Check sheet for the modelled part. Datum: model origin and axes. Units: mm. A direction names the side the tool comes from. Give positions to 0.01 mm unless a question says otherwise; leave off trailing zeros. Order: outer loops, then holes, each group sorted by start corner. A loop starts at its lowest first (then second) coordinate and runs counter-clockwise, first axis right, second up. Notation, with made-up numbers: (-40, -32) -> (-12, -32) arc R23 ccw to (-12, 6) -> close; hole circle Ø11 at (68.5, 36.25). An arc over 180 degrees is marked (long way). One line per question, with ' | ' between items.
```python
from build123d import *

# Parameters (mm, degrees)
CYLINDER_R           = 2.15
CYLINDER_DEPTH       = 50
CYLINDER_PITCH_ANGLE = 90
BOX002_W             = 14
BOX002_H             = 11
BOX002_DEPTH         = 20.5
CHAMFER_SIZE         = 4
FILLET001_R          = 5
BOX003_W             = 14
BOX003_H             = 25
BOX003_DEPTH         = 4
BOX003_ROLL_ANGLE    = -15
BOX004_W             = 14
BOX004_H             = 2.5
BOX004_DEPTH         = 5
POCKET006_DEPTH      = 15
BOX005003_W          = 42
BOX005003_H          = 6
BOX005003_DEPTH      = 25
SKETCH009_R          = 11
SKETCH009_R_2        = 1.75
POCKET009_DEPTH      = 6
SKETCH010_W          = 62.382877
SKETCH010_H          = 25.148186
POCKET010_DEPTH      = 6
BOX005002_W          = 13.8
BOX005002_H          = 6
BOX005002_DEPTH      = 42
CHAMFER002_SIZE      = 13
FILLET003_R          = 4
FILLET004_R          = 2
SKETCH011_R          = 2.95
POCKET011_DEPTH      = 4


with BuildPart() as cylinder:
    # Cylinder → Cylinder (new body)
    with BuildSketch(Plane.XY):
        Circle(CYLINDER_R)
    extrude(amount=CYLINDER_DEPTH)


with BuildPart() as cylinder_1:
    # Cylinder pitch: moved
    add(cylinder.part.rotate(Axis((0, 0, 0), (0, 1, 0)), CYLINDER_PITCH_ANGLE))


with BuildPart() as cylinder_2:
    # Cylinder placement: moved
    add(cylinder_1.part.moved(Location((31, -6, 12.9))))


with BuildPart() as fillet001:
    # Box002 → Box002 (new body)
    with BuildSketch(Plane(origin=(52, -12, -3), x_dir=(1, 0, 0), z_dir=(0, 0, 1))):
        with Locations((7, 5.5)):
            Rectangle(BOX002_W, BOX002_H)
    extrude(amount=BOX002_DEPTH)

    # Chamfer
    chamfer_edges = [fillet001.edges().sort_by_distance(p)[0] for p in [
        (59, -1, -3),
    ]]
    chamfer(chamfer_edges, length=CHAMFER_SIZE)

    # Fillet001
    fillet001_edges = [fillet001.edges().sort_by_distance(p)[0] for p in [
        (59, -1, 17.5),
    ]]
    fillet(fillet001_edges, radius=FILLET001_R)


with BuildPart() as cube002:
    # Box003 → Box003 (new body)
    with BuildSketch(Plane.XY):
        with Locations((7, 12.5)):
            Rectangle(BOX003_W, BOX003_H)
    extrude(amount=BOX003_DEPTH)


with BuildPart() as cube002_1:
    # Box003 roll: moved
    add(cube002.part.rotate(Axis((0, 0, 0), (1, 0, 0)), BOX003_ROLL_ANGLE))


with BuildPart() as cube002_2:
    # Box003 placement: moved
    add(cube002_1.part.moved(Location((52, -12, -3))))


with BuildPart() as obj1:
    # Box004 → Box004 (new body)
    with BuildSketch(Plane(origin=(52, -12, 14), x_dir=(1, 0, 0), z_dir=(0, 0, 1))):
        with Locations((7, 1.25)):
            Rectangle(BOX004_W, BOX004_H)
    extrude(amount=BOX004_DEPTH)

    # Fusion: union Fillet001, Cube002
    add(fillet001.part)
    add(cube002_2.part)

    # Cut001: cut Cylinder
    add(cylinder_2.part, mode=Mode.SUBTRACT)

    # Sketch006 → Pocket006 (cut)
    with BuildSketch(Plane.YZ.offset(66)):
        Polygon((13.183422, -5.606773), (-4.041064, -0.991486), (-0.407217, 12.570217), align=None)
    extrude(amount=-POCKET006_DEPTH, mode=Mode.SUBTRACT)


with BuildPart() as pocket010:
    # Box005003 → Box005003 (new body)
    with BuildSketch(Plane(origin=(52.2, -15.5, -42), x_dir=(1, 0, 0), z_dir=(0, 0, 1))):
        with Locations((21, 3)):
            Rectangle(BOX005003_W, BOX005003_H)
    extrude(amount=BOX005003_DEPTH)

    # Sketch009 → Pocket009 (cut)
    with BuildSketch(Plane(origin=(52.2, -9.5, -42), x_dir=(-1, 0, 0), z_dir=(0, 1, 0))):
        with Locations((-21, 1.5)):
            Circle(SKETCH009_R)
        with Locations((-36.5, 17)):
            Circle(SKETCH009_R_2)
        with Locations((-5.5, 17)):
            Circle(SKETCH009_R_2)
    extrude(amount=-POCKET009_DEPTH, mode=Mode.SUBTRACT)

    # Sketch010 → Pocket010 (cut)
    with BuildSketch(Plane(origin=(52.2, -9.5, -42), x_dir=(-1, 0, 0), z_dir=(0, 1, 0))):
        with Locations((-19.46246, -4.449775)):
            Rectangle(SKETCH010_W, SKETCH010_H)
    extrude(amount=-POCKET010_DEPTH, mode=Mode.SUBTRACT)


with BuildPart() as pocket011:
    # Box005002 → Box005002 (new body)
    with BuildSketch(Plane(origin=(52.2, -15.5, -21), x_dir=(1, 0, 0), z_dir=(0, 0, 1))):
        with Locations((6.9, 3)):
            Rectangle(BOX005002_W, BOX005002_H)
    extrude(amount=BOX005002_DEPTH)

    # Fusion005: union obj1, Pocket010
    add(obj1.part)
    add(pocket010.part)

    # Chamfer002
    chamfer002_edges = [pocket011.edges().sort_by_distance(p)[0] for p in [
        (66, -12.5, -17),
    ]]
    chamfer(chamfer002_edges, length=CHAMFER002_SIZE)

    # Fillet003
    fillet003_edges = [pocket011.edges().sort_by_distance(p)[0] for p in [
        (94.2, -12.5, -17),
        (94.2, -12.5, -33.875682),
        (52.2, -12.5, -33.875682),
    ]]
    fillet(fillet003_edges, radius=FILLET003_R)

    # Fillet004
    fillet004_edges = [pocket011.edges().sort_by_distance(p)[0] for p in [
        (59.1, -9.5, 21),
    ]]
    fillet(fillet004_edges, radius=FILLET004_R)

    # Sketch011 → Pocket011 (cut)
    with BuildSketch(Plane(origin=(0, -9.5, 0), x_dir=(-1, 0, 0), z_dir=(0, 1, 0))):
        with Locations((-88.7, -25)):
            Circle(SKETCH011_R)
        with Locations((-57.7, -25)):
            Circle(SKETCH011_R)
    extrude(amount=-POCKET011_DEPTH, mode=Mode.SUBTRACT)


solid = pocket011.part
```
Q1. Section check A-A (x = 88.7). Enter the section's corners in (y, z).
Result sheet:
outline: (-15.5, -33.88) -> (-9.5, -33.88) -> (-9.5, -27.95) -> (-13.5, -27.95) -> (-13.5, -26.75) -> (-15.5, -26.75) -> close; (-15.5, -23.25) -> (-13.5, -23.25) -> (-13.5, -22.05) -> (-9.5, -22.05) -> (-9.5, -17) -> (-15.5, -17) -> close
Q2. Access from +Z, -Z, +X, -X, +Y, -Y to the whole of each face (thin tool, end or side, straight path). Record for faces 1 (the face through (52, -5, 5)), 2 (the face through (85, -12, -17)), 3 (the face through (66, -8, 6)), 4 (the face through (94.2, -13, -25)), 5 (the face through (59, -1, 11)).
Result sheet:
face 1: +Z, -Z, -X, +Y, -Y | face 2: +Z, +X, +Y, -Y | face 3: +Z, +X, +Y | face 4: +Z, -Z, +X, +Y, -Y | face 5: +Z, +X, -X, +Y
Q3. Thickness scan on line 1 (Z direction, x = 57.7, y = -14.55); line 2 (Z direction, x = 88.7, y = -14.45); line 3 (Y direction, x = 73.5, z = -26). Record the ranges inside material, lowest first.
Result sheet:
line 1: z = -33.88 to -26.75, -23.25 to 21 | line 2: z = -33.88 to -26.75, -23.25 to -17 | line 3: y = -15.5 to -9.5
Q4. Depth check by flat-ended pin: pin 1 Ø1.8 at (x, y) = (61, -8.5) entering from +Z; pin 2 Ø9.5 at (x, z) = (57.7, -25) entering from +Y; pin 3 Ø2.5 at (x, z) = (59.5, 11) entering from +Y; pin 4 Ø3.5 at (y, z) = (-6, 12.9) entering from -X. Enter the tip coordinate at first touch or a pass-through.
Result sheet:
pin 1: stops at z = 17.5 | pin 2: stops at y = -9.5 | pin 3: stops at y = -1 | pin 4: passes through
Q5. Section check C-C (z = -25). Enter the section's corners in (x, y), and give its area (3 significant figures).
Result sheet:
outline: (52.2, -15.5) -> (55.95, -15.5) -> (55.95, -13.5) -> (54.75, -13.5) -> (54.75, -9.5) -> (52.2, -9.5) -> close; (59.45, -15.5) -> (86.95, -15.5) -> (86.95, -13.5) -> (85.75, -13.5) -> (85.75, -9.5) -> (60.65, -9.5) -> (60.65, -13.5) -> (59.45, -13.5) -> close; (90.45, -15.5) -> (94.2, -15.5) -> (94.2, -9.5) -> (91.65, -9.5) -> (91.65, -13.5) -> (90.45, -13.5) -> close | area: 191 mm2
Q6. Section check D-D (x = 68). Enter the section's corners in (y, z), and give its area (3 significant figures).
Result sheet:
outline: (-15.5, -30.81) -> (-9.5, -30.81) -> (-9.5, -6) -> (-15.5, -6) -> close | area: 149 mm2
Q7. Mould release check, pull along Y, two halves, no side actions. Record for faces 6 (the face through (53.34, -12.54, -32.67)), 7 (the face through (58.9, 0.24, -6.28)), 8 (the face through (58.902, 12.659, -7.566)): pulls with the +Y half, pulls with the -Y half, needs draft (parallel to the pull), parting line crosses it, or undercut.
Result sheet:
face 6: needs draft | face 7: undercut | face 8: pulls with the +Y half
Q8. Section check B-B (x = 57.7). Enter the section's corners in (y, z), and give its area (3 significant figures).
Result sheet:
outline: (-15.5, -33.88) -> (-9.5, -33.88) -> (-9.5, -27.95) -> (-13.5, -27.95) -> (-13.5, -26.75) -> (-15.5, -26.75) -> close; (-15.5, -23.25) -> (-13.5, -23.25) -> (-13.5, -22.05) -> (-9.5, -22.05) -> (-9.5, -3.67) -> (12.15, -9.47) -> (13.18, -5.61) -> (-4.04, -0.99) -> (-1, 10.36) -> (-1, 12.5) arc R5 ccw to (-6, 17.5) -> (-9.5, 17.5) -> (-9.5, 19) arc R2 ccw to (-11.5, 21) -> (-15.5, 21) -> close; hole circle Ø4.3 at (-6, 12.9) | area: 506 mm2
